Could you check a few things on this drawing? It's one solid part, dimensions in mm from its lowest x, y, z. Give positions to 0.01 mm unless a question says otherwise; leave off trailing zeros. Loops run counter-clockwise (first coordinate to the right, second up) from the corner with the lowest first, then second, coordinate; pieces in that order, holes last. Notation, with made-up numbers: (49.5, 86.5) - (61.5, 86.5) arc R22 ccw to (61.5, 110.5) - close; hole circle Ø8 at (53, 80). An arc over 180 degrees is marked (long way). Return JSON: item names as keys, results as strings. Group by question number.
(1) If we section it at A-A (y = 10.75): Please give me the cut outline in (x, z), then the cut area to 3 significant figures.
(2) I need wall thicknesses on probe 1 along Z at (x, y) = (4, 20); probe 2 along Y at (x, z) = (3.9, 4). Which ranges of each line are inside material? Lowest first, please. Write a range as [from, to].
(3) For P1, Ø1.5, axis at x = 6, y = 6.5, coming from the +Z side; P2, Ø4, axis at x = 3.9, z = 3.9, coming from the +Y side; P3, Ø1.5, axis at y = 16, z = 1.5, coming from the +X side, each with a flat end and sliding along its axis, tell me the tip position at first contact or that it passes through.
(4) If we mould it in two halves opening along Y, with no side actions, what happens to the marked faces 1, 2, 3 and 4? For each: released by +Y, released by -Y, zero draft, split by the parting line, or undercut.
(5) If we section it at B-B (y = 5): Please give me the cut outline in (x, z).
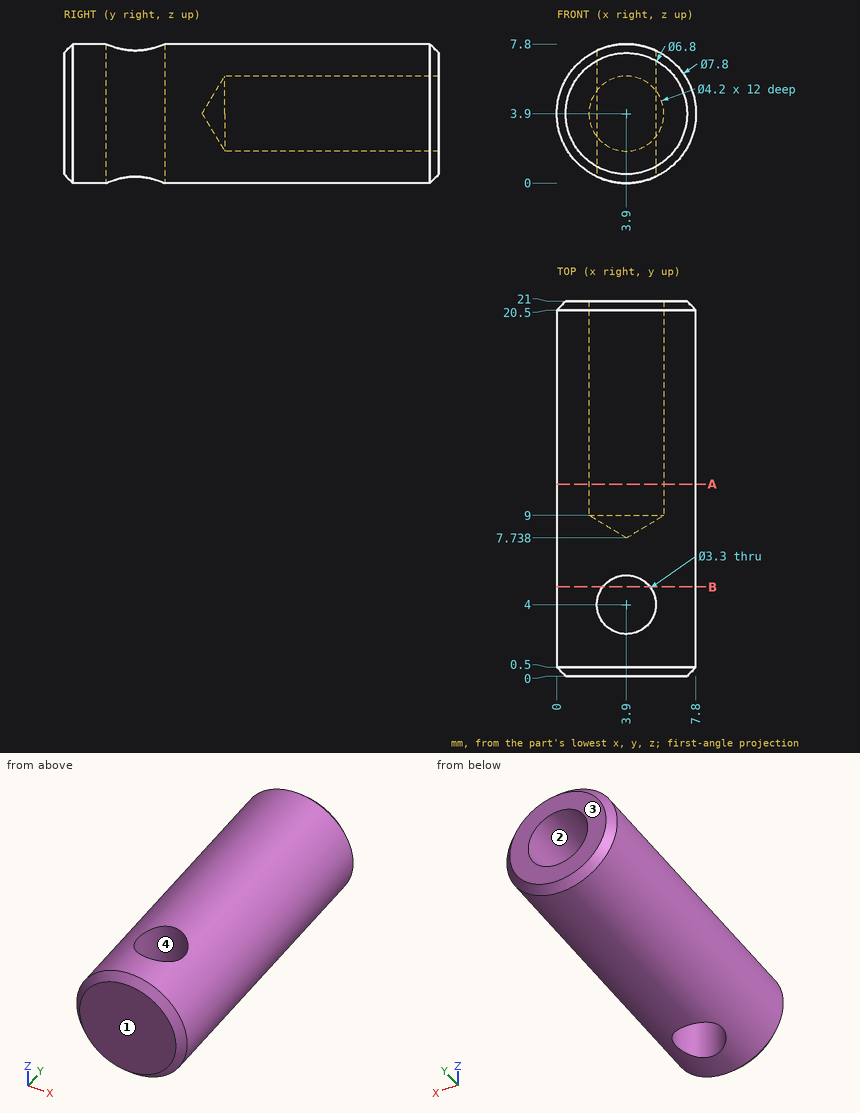
Values:
{
 "1": {"outline": "circle Ø7.8 at (3.9, 3.9); hole circle Ø4.2 at (3.9, 3.9)", "area": "33.9 mm2"},
 "2": {"probe 1": "[0, 1.8], [6, 7.8]", "probe 2": "[0, 2.35], [5.65, 7.8]"},
 "3": {"P1": "z = 7.56", "P2": "y = 8.94", "P3": "x = 7.43"},
 "4": {"face 1": "released by -Y", "face 2": "zero draft", "face 3": "released by +Y", "face 4": "undercut"},
 "5": {"outline": "(2.59, 0.23) - (2.59, 7.57) arc R3.9 ccw to start; (5.21, 0.23) arc R3.9 ccw to (5.21, 7.57) - close"}
}
